```python
from build123d import *

# Parameters (mm, degrees)
SKETCH1_R           = 12.7
BOSS_EXTRUDE1_DEPTH = 12.7
SKETCH2_R           = 3.175
CUT_EXTRUDE1_DEPTH  = 12.7


with BuildPart() as part:
    # Sketch1 → Boss-Extrude1 (new body)
    with BuildSketch(Plane(origin=(0, 0, 0), x_dir=(1, 0, 0), z_dir=(0, 1, 0))):
        with BuildLine():
            Line((11.636850036, 9.840798811), (27.196051224, 25.4))
            Line((27.196051224, 25.4), (150.603948776, 25.4))
            Line((150.603948776, 25.4), (166.163149964, 9.840798811))
            ThreePointArc((166.163149964, 9.840798811), (188.576307345, -10.776307345), (167.959201189, 11.636850036))
            Line((167.959201189, 11.636850036), (151.656051224, 27.94))
            Line((151.656051224, 27.94), (26.143948776, 27.94))
            Line((26.143948776, 27.94), (9.840798811, 11.636850036))
            ThreePointArc((9.840798811, 11.636850036), (-10.776307345, -10.776307345), (11.636850036, 9.840798811))
        make_face()
        with Locations(Location((0, 0, 0), (0, 0, 270))):
            Circle(SKETCH1_R, mode=Mode.SUBTRACT)
        with Locations(Location((177.8, 0, 0), (0, 0, 270))):
            Circle(SKETCH1_R, mode=Mode.SUBTRACT)
    extrude(amount=BOSS_EXTRUDE1_DEPTH)

    # Sketch2 → Cut-Extrude1 (cut)
    with BuildSketch(Plane.XY.offset(-25.4)):
        with Locations((47.64999995, 6.35)):
            Circle(SKETCH2_R)
        with Locations((130.15000005, 6.35)):
            Circle(SKETCH2_R)
    extrude(amount=-CUT_EXTRUDE1_DEPTH, mode=Mode.SUBTRACT)


solid = part.part
```
Geometry: final body of the model. Coordinates: model frame, mm. A direction names the side the tool comes from. Round coordinates to 2 decimals unless told otherwise and drop trailing zeros. Write each loop counter-clockwise with the first axis right and the second up, starting at its lowest first coordinate (ties: lowest second). Pieces come first, ordered by that corner, then holes.
Item 1: Pin query (flat end, axial travel): P1, Ø5, axis at y = 10, z = 8, coming from the +X side; P2, Ø20.5, axis at x = 0, z = 0, coming from the -Y side; P3, Ø1, axis at x = 95.5, y = 6, coming from the +Z side; P4, Ø3, axis at y = 8, z = -13.5, coming from the -X side. Return the tip coordinate at first contact, or that it passes through.
Item 2: Section query A-A (y = 6.35). Return loops of the section in (x, z) (3 decimals).
Item 3: Section query B-B (x = 0). Return loops of the section in (y, z).
Item 4: Mould query, pull axis Y, two halves, no side actions, for faces 1 (the face through (50.68, 7.3, -26.65)), 2 (the face through (159.922, 6.261, -19.674)), 3 (the face through (88, 0, -26)). Classes: +Y half, -Y half, draft (parallel to the pull), parting line (faces both ways), or undercut.
Item 5: Section query D-D (x = 47.65). Return loops of the section in (y, z) (3 decimals), plus the area to 3 significant figures.
Item 6: Material intervals for L1, parallel to X at y = 6.5, z = 0; L2, parallel to Y at x = 47.65, z = -26.1 (3 decimals); L3, parallel to X at y = 8, z = 7.5, sorted ascending.
Item 7: Set-up query: faces 4 (the face through (88, 6, -25.4)), 5 (the face through (19.308, 6.261, -17.511)), 6 (the face through (18.106, 6.261, -19.903)). Return all of +Z, -Z, +X, -X, +Y, -Y with unobstructed straight access to the full face (end or side cutting, diameter ignored); none if empty.
Item 8: Section query C-C (z = 0). Return loops of the section in (x, y).
Completed:
1. P1: stops at x = 192.01
1. P2: passes through
1. P3: stops at z = -25.4
1. P4: stops at x = -9.39
2. outline: (9.841, -11.637) - (26.144, -27.94) - (44.475, -27.94) - (44.475, -25.4) - (27.196, -25.4) - (11.637, -9.841) arc R15.24 ccw (long way) to start; (50.825, -27.94) - (126.975, -27.94) - (126.975, -25.4) - (50.825, -25.4) - close; (133.325, -27.94) - (151.656, -27.94) - (167.959, -11.637) arc R15.24 ccw (long way) to (166.163, -9.841) - (150.604, -25.4) - (133.325, -25.4) - close; hole circle Ø25.4 at (0, 0); hole circle Ø25.4 at (177.8, 0)
3. outline: (0, -15.24) - (12.7, -15.24) - (12.7, -12.7) - (0, -12.7) - close; (0, 12.7) - (12.7, 12.7) - (12.7, 15.24) - (0, 15.24) - close
4. face 1: undercut
4. face 2: draft
4. face 3: -Y half
5. outline: (0, -27.94) - (3.175, -27.94) - (3.175, -25.4) - (0, -25.4) - close; (9.525, -27.94) - (12.7, -27.94) - (12.7, -25.4) - (9.525, -25.4) - close
5. area: 16.1 mm2
6. L1: x = -15.24 to -12.7, 12.7 to 15.24, 162.56 to 165.1, 190.5 to 193.04
6. L2: y = 0 to 3.175, 9.525 to 12.7
6. L3: x = -13.27 to -10.25, 10.25 to 13.27, 164.53 to 167.55, 188.05 to 191.07
7. face 4: +Z, +Y, -Y
7. face 5: +Y, -Y
7. face 6: -Z, +Y, -Y
8. outline: (-15.24, 0) - (-12.7, 0) - (-12.7, 12.7) - (-15.24, 12.7) - close; (12.7, 0) - (15.24, 0) - (15.24, 12.7) - (12.7, 12.7) - close; (162.56, 0) - (165.1, 0) - (165.1, 12.7) - (162.56, 12.7) - close; (190.5, 0) - (193.04, 0) - (193.04, 12.7) - (190.5, 12.7) - close
